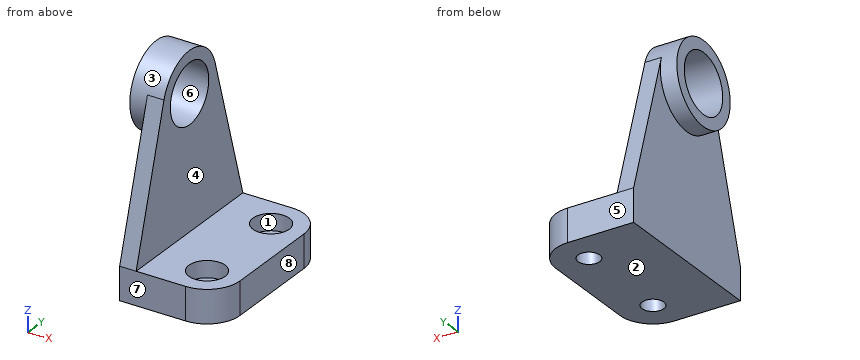
from build123d import *

# Parameters (mm, degrees)
SKETCH_1_W                = 30
SKETCH_1_H                = 50
EXTRUDE_2_DEPTH           = 10
EXTRUDE_3_DEPTH           = 5
EXTRUDE_4_DEPTH           = 5
EXTRUDE_4_DEPTH_BACK      = 5
SKETCH_2_3_R              = 12.5
SKETCH_2_3_R_2            = 9
FILLET_1_R                = 10
HOLE_WIZARD_1_D           = 6.6
HOLE_WIZARD_1_CBORE_D     = 11
HOLE_WIZARD_1_CBORE_DEPTH = 5


with BuildPart() as part:
    # Sketch 1 → Extrude 2 (new body)
    with BuildSketch(Plane.XY):
        Rectangle(SKETCH_1_W, SKETCH_1_H)
    extrude(amount=EXTRUDE_2_DEPTH)

    # Sketch 2 → Extrude 3 (add)
    with BuildSketch(Plane.ZY.offset(15)):
        with BuildLine():
            Line((10, 25), (10, -25))
            Line((10, -25), (53.579145154, -11.976632246))
            ThreePointArc((53.579145154, -11.976632246), (37.5, 0), (53.579145154, 11.976632246))
            Line((53.579145154, 11.976632246), (10, 25))
        make_face()
    extrude(amount=-EXTRUDE_3_DEPTH)

    # Sketch 2_3 → Extrude 4 (add, two sides: drawn at the far end of the back side and taken through both)
    with BuildSketch(Plane.ZY.offset(15).offset(-EXTRUDE_4_DEPTH_BACK)):
        with Locations((50, 0)):
            Circle(SKETCH_2_3_R)
        with Locations((50, 0)):
            Circle(SKETCH_2_3_R_2, mode=Mode.SUBTRACT)
    extrude(amount=EXTRUDE_4_DEPTH + EXTRUDE_4_DEPTH_BACK)

    # Fillet 1
    fillet_1_edges = [part.edges().sort_by_distance(p)[0] for p in [
        (15, -25, 5),
        (15, 25, 5),
    ]]
    fillet(fillet_1_edges, radius=FILLET_1_R)

    # Hole Wizard 1 (through all)
    with Locations(Plane.XY.offset(10)):
        with Locations((5, -15), (5, 15)):
            CounterBoreHole(HOLE_WIZARD_1_D / 2, HOLE_WIZARD_1_CBORE_D / 2, HOLE_WIZARD_1_CBORE_DEPTH)


solid = part.part
Check sheet for the modelled part. Datum: model origin and axes. Units: mm. Face numbers are marked on the shaded views. A direction names the side the tool comes from. Round coordinates to 2 decimals unless told otherwise and drop trailing zeros. Order: outer loops, then holes, each group sorted by start corner. A loop starts at its lowest first (then second) coordinate and runs counter-clockwise, first axis right, second up.
Q1. Depth check by flat-ended pin: P1, Ø6, axis at x = 5, y = 15, coming from the +Z side; P2, Ø14.5, axis at x = 5, y = -15, coming from the +Z side; P3, Ø3.5, axis at x = 7.5, y = -16.5, coming from the +Z side; P4, Ø1.5, axis at y = -12, z = 22, coming from the +X side. Enter the tip coordinate at first touch or a pass-through.
Filled sheet:
P1: passes through
P2: stops at z = 10
P3: stops at z = 5
P4: stops at x = -10
Q2. Scan lines: L1, parallel to Z at x = 11.5, y = -10.5; L2, parallel to Y at x = -10.5, z = 58; L3, parallel to X at y = -6, z = 24.5. Record each from-to range of solid material in increasing order.
Filled sheet:
L1: z = 0 to 10
L2: y = -9.6 to -4.12, 4.12 to 9.6
L3: x = -15 to -10
Q3. Cross-section at B-B, the plane z = 50. Enter the section's corners in (x, y), plus the area to 3 significant figures.
Filled sheet:
outline: (-20, -12.5) - (-15, -12.5) - (-15, -13.05) - (-10, -13.05) - (-10, -9) - (-20, -9) - close; (-20, 9) - (-10, 9) - (-10, 13.05) - (-15, 13.05) - (-15, 12.5) - (-20, 12.5) - close
area: 75.5 mm2
Q4. Set-up check for the marked faces 1, 2, 3, 4 and 5: record each of +Z, -Z, +X, -X, +Y, -Y from which the full face is reachable in a straight line by a thin tool's end or side.
Filled sheet:
face 1: +Z
face 2: -Z, +X, -X, +Y, -Y
face 3: -X
face 4: +Z, +X, +Y, -Y
face 5: +Z, -Z, +X, -X, +Y
Q5. Cross-section at D-D, the plane y = 17. Enter the section's corners in (x, z), plus the area to 3 significant figures.
Filled sheet:
outline: (-15, 0) - (2.38, 0) - (2.38, 5) - (-0.12, 5) - (-0.12, 10) - (-10, 10) - (-10, 36.77) - (-15, 36.77) - close; (7.62, 0) - (14.8, 0) - (14.8, 10) - (10.12, 10) - (10.12, 5) - (7.62, 5) - close
area: 354 mm2
Q6. Cross-section at C-C, the plane x = 9.5. Enter the section's corners in (y, z), plus the area to 3 significant figures.
Filled sheet:
outline: (-23.93, 0) - (23.93, 0) - (23.93, 10) - (18.16, 10) - (18.16, 5) - (11.84, 5) - (11.84, 10) - (-11.84, 10) - (-11.84, 5) - (-18.16, 5) - (-18.16, 10) - (-23.93, 10) - close
area: 415 mm2
Q7. Draft check along Y on the marked faces 6, 7 and 8. Enter one of: pulls with the +Y half, pulls with the -Y half, needs draft (parallel to the pull), parting line crosses it, or undercut.
Filled sheet:
face 6: undercut
face 7: pulls with the -Y half
face 8: needs draft
Q8. Cross-section at A-A, the plane y = 0. Enter the section's corners in (x, z), plus the area to 4 significant figures.
Filled sheet:
outline: (-20, 37.5) - (-15, 37.5) - (-15, 0) - (15, 0) - (15, 10) - (-10, 10) - (-10, 41) - (-20, 41) - close; (-20, 59) - (-10, 59) - (-10, 62.5) - (-20, 62.5) - close
area: 507.5 mm2
